```python
from build123d import *

# Parameters (mm, degrees)
CROQUIS5_R              = 2.552588688
SALIENTE_EXTRUIR4_DEPTH = 8
CORTAR_EXTRUIR2_START   = -5
CROQUIS6_R              = 2.552588688
CORTAR_EXTRUIR2_DEPTH   = 5
CROQUIS7_W              = 7
CROQUIS7_H              = 13
CORTAR_EXTRUIR3_DEPTH   = 6
CROQUIS8_W              = 15
CROQUIS8_H              = 30
CORTAR_EXTRUIR4_DEPTH   = 10
CROQUIS9_R              = 4.05
SALIENTE_EXTRUIR5_DEPTH = 3
CROQUIS10_R             = 2.1
CORTAR_EXTRUIR5_DEPTH   = 3


with BuildPart() as part:
    # Croquis5 → Saliente-Extruir4 (new body)
    with BuildSketch(Plane.XY):
        with BuildLine():
            Line((-12.912379316, 50.582104264), (38.083380168, 50.582104264))
            Line((38.083380168, 50.582104264), (38.083380168, 54.811507329))
            ThreePointArc((38.083380168, 54.811507329), (38.888836519, 56.756050977), (40.833380168, 57.561507329))
            Line((40.833380168, 57.561507329), (43.833380168, 57.561507329))
            ThreePointArc((43.833380168, 57.561507329), (45.777923816, 56.756050977), (46.583380168, 54.811507329))
            Line((46.583380168, 54.811507329), (46.583380168, 40.332104264))
            ThreePointArc((46.583380168, 40.332104264), (45.777923816, 38.387560616), (43.833380168, 37.582104264))
            Line((43.833380168, 37.582104264), (40.833380168, 37.582104264))
            ThreePointArc((40.833380168, 37.582104264), (38.888836519, 38.387560616), (38.083380168, 40.332104264))
            Line((38.083380168, 40.332104264), (38.083380168, 44.482104264))
            Line((38.083380168, 44.482104264), (-12.912379316, 44.482104264))
            ThreePointArc((-12.912379316, 44.482104264), (-19.776162486, 47.532104264), (-12.912379316, 50.582104264))
        make_face()
        with Locations((-15.666619832, 47.532104264)):
            Circle(CROQUIS5_R, mode=Mode.SUBTRACT)
    extrude(amount=SALIENTE_EXTRUIR4_DEPTH)

    # Croquis6 → Cortar-Extruir2 (cut)
    with BuildSketch(Plane.XY.offset(8).offset(CORTAR_EXTRUIR2_START)):
        with BuildLine():
            Line((-12.912379316, 50.582104264), (38.083380168, 50.582104264))
            Line((38.083380168, 50.582104264), (38.083380168, 53.082104264))
            Line((38.083380168, 53.082104264), (39.583380168, 53.082104264))
            Line((39.583380168, 53.082104264), (39.583380168, 42.082104264))
            Line((39.583380168, 42.082104264), (38.083380168, 42.082104264))
            Line((38.083380168, 42.082104264), (38.083380168, 44.482104264))
            Line((38.083380168, 44.482104264), (-12.912379316, 44.482104264))
            ThreePointArc((-12.912379316, 44.482104264), (-19.776162486, 47.532104264), (-12.912379316, 50.582104264))
        make_face()
        with Locations((-15.666619832, 47.532104264)):
            Circle(CROQUIS6_R, mode=Mode.SUBTRACT)
    extrude(amount=CORTAR_EXTRUIR2_DEPTH, mode=Mode.SUBTRACT)

    # Croquis7 → Cortar-Extruir3 (cut)
    with BuildSketch(Plane.XY.offset(8)):
        with Locations((43.083380168, 47.582104264)):
            Rectangle(CROQUIS7_W, CROQUIS7_H)
    extrude(amount=-CORTAR_EXTRUIR3_DEPTH, mode=Mode.SUBTRACT)

    # Croquis8 → Cortar-Extruir4 (cut)
    with BuildSketch(Plane(origin=(0, 0, 0), x_dir=(-1, 0, 0), z_dir=(0, 0, -1))):
        with Locations((12.276162486, 38.194032094)):
            Rectangle(CROQUIS8_W, CROQUIS8_H)
    extrude(amount=-CORTAR_EXTRUIR4_DEPTH, mode=Mode.SUBTRACT)

    # Croquis9 → Saliente-Extruir5 (add)
    with BuildSketch(Plane(origin=(0, 0, 0), x_dir=(-1, 0, 0), z_dir=(0, 0, -1))):
        with Locations((4.776162486, 47.532104264)):
            Circle(CROQUIS9_R)
    extrude(amount=-SALIENTE_EXTRUIR5_DEPTH)

    # Croquis10 → Cortar-Extruir5 (cut)
    with BuildSketch(Plane(origin=(0, 0, 0), x_dir=(-1, 0, 0), z_dir=(0, 0, -1))):
        with Locations((4.776162486, 47.532104264)):
            Circle(CROQUIS10_R)
    extrude(amount=-CORTAR_EXTRUIR5_DEPTH, mode=Mode.SUBTRACT)


solid = part.part
```
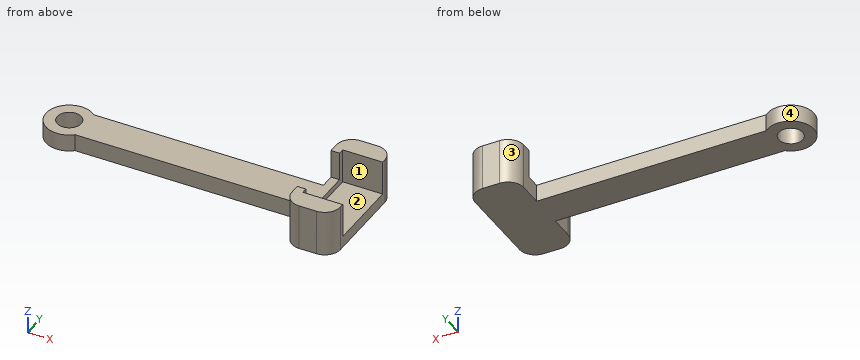
Design review of the part built by this model. Coordinates are the model's own, in mm. Face numbers are marked on the shaded views. Coordinates: 2 decimals unless noted, no trailing zeros. Order: outer loops, then holes, each group sorted by start corner. A loop starts at its lowest first (then second) coordinate and runs counter-clockwise, first axis right, second up.
1) Clearance check with flat-ended pins moving along their axes: pin 1 (1.5 mm diameter, centred on x = 10, z = 2, fed in from +Y); pin 2 (3.5 mm diameter, centred on x = 6.5, y = 45.5, fed in from +Z); pin 3 (4 mm diameter, centred on y = 43.5, z = 2, fed in from -X). State where each tip first meets the part, or that it passes through.
2) Take a section at D-D, the plane z = 1.25. Give the boundary of the cut face in (x, y), and give its area (3 significant figures).
3) Mouldability with a two-part tool opening along Y and no side actions: class the marked faces 1, 2, 3 and 4 as +Y half, -Y half, draft (parallel to the pull), parting line (faces both ways), or undercut.
4) Take a section at C-C, the plane y = 46.5. Give the boundary of the cut face in (x, z), and give its area (3 significant figures).
5) Take a section at B-B, the plane x = 41.5. Give the boundary of the cut face in (y, z).
6) Wall thickness on line 1 along X through (y, z) = (42.5, 2.5); line 2 along Y through (x, z) = (41.5, 6); line 3 along Z through (x, y) = (-4.5, 43.75): over which ranges is each line inside the solid? List them lowest first.
7) Take a section at A-A, the plane z = 6.25. Give the boundary of the cut face in (x, y), and give its area (3 significant figures).
Returned:
1. pin 1: stops at y = 50.58
1. pin 2: stops at z = 3
1. pin 3: stops at x = -8.28
2. outline: (-2.11, 44.48) - (38.08, 44.48) - (38.08, 40.33) arc R2.75 ccw to (40.83, 37.58) - (43.83, 37.58) arc R2.75 ccw to (46.58, 40.33) - (46.58, 54.81) arc R2.75 ccw to (43.83, 57.56) - (40.83, 57.56) arc R2.75 ccw to (38.08, 54.81) - (38.08, 50.58) - (-2.11, 50.58) arc R4.05 ccw (long way) to start; hole circle Ø4.2 at (-4.78, 47.53)
2. area: 440 mm2
3. face 1: undercut
3. face 2: undercut
3. face 3: +Y half
3. face 4: parting line
4. outline: (-8.69, 0) - (-6.61, 0) - (-6.61, 3) - (-8.69, 3) - close; (-2.95, 0) - (46.58, 0) - (46.58, 2) - (39.58, 2) - (39.58, 3) - (-2.95, 3) - close
4. area: 148 mm2
5. outline: (37.58, 0) - (57.56, 0) - (57.56, 8) - (54.08, 8) - (54.08, 2) - (41.08, 2) - (41.08, 8) - (37.58, 8) - close
6. line 1: x = 38.08 to 39.58
6. line 2: y = 37.58 to 41.08, 54.08 to 57.56
6. line 3: z = 0 to 3
7. outline: (38.08, 40.33) arc R2.75 ccw to (40.83, 37.58) - (43.83, 37.58) arc R2.75 ccw to (46.58, 40.33) - (46.58, 41.08) - (39.58, 41.08) - (39.58, 42.08) - (38.08, 42.08) - close; (38.08, 53.08) - (39.58, 53.08) - (39.58, 54.08) - (46.58, 54.08) - (46.58, 54.81) arc R2.75 ccw to (43.83, 57.56) - (40.83, 57.56) arc R2.75 ccw to (38.08, 54.81) - close
7. area: 55.8 mm2
